from build123d import *

# Parameters (mm, degrees)
SKETCH1_R           = 20
BOSS_EXTRUDE1_DEPTH = 70
SKETCH2_R           = 15
CUT_EXTRUDE1_DEPTH  = 70
SKETCH3_R           = 2.5
CUT_EXTRUDE2_DEPTH  = 53


with BuildPart() as part:
    # Sketch1 → Boss-Extrude1 (new body)
    with BuildSketch(Plane.XY):
        Circle(SKETCH1_R)
    extrude(amount=BOSS_EXTRUDE1_DEPTH)

    # Sketch2 → Cut-Extrude1 (cut)
    with BuildSketch(Plane.XY.offset(70)):
        Circle(SKETCH2_R)
    extrude(amount=-CUT_EXTRUDE1_DEPTH, mode=Mode.SUBTRACT)

    # Sketch3 → Cut-Extrude2 (cut)
    with BuildSketch(Plane(origin=(20, 0, 0), x_dir=(0, 0, -1), z_dir=(1, 0, 0))):
        with Locations((-25, 0)):
            Circle(SKETCH3_R)
    extrude(amount=-CUT_EXTRUDE2_DEPTH, mode=Mode.SUBTRACT)


solid = part.part
The listing builds one solid part. Answer for the finished solid, in the listing's coordinates (mm). Coordinates: 2 decimals unless noted, no trailing zeros. Write each loop counter-clockwise with the first axis right and the second up, starting at its lowest first coordinate (ties: lowest second). Pieces come first, ordered by that corner, then holes. Notation, with made-up numbers: M 55,50.5 L 91,50.5 A15 cw 91,66.5 Z; hole C 52,18.25 d8. An arc over 180 degrees is marked long. Write each question's results on one line, items separated by ' | '.
Item 1: For a pull along Z with two mould halves and no side action, classify faces 1 (the face through (-17.4, 0.1, 27.5)), 2 (the face through (17.4, 0.1, 27.5)), 3 (the face through (3, 15, 70)), 4 (the face through (19.076, 6.007, 34.51)) as released by +Z, released by -Z, zero draft, split by the parting line, or undercut.
Answer below:
face 1: undercut | face 2: undercut | face 3: released by +Z | face 4: zero draft
Item 2: The part is cut by section B-B on y = 0. Determine the outline of the cut face in (x, z).
Answer below:
outline: M -20,0 L -15,0 L -15,22.5 L -20,22.5 Z; M -20,27.5 L -15,27.5 L -15,70 L -20,70 Z; M 15,0 L 20,0 L 20,22.5 L 15,22.5 Z; M 15,27.5 L 20,27.5 L 20,70 L 15,70 Z
Item 3: The part is cut by section C-C on x = 12. Determine the outline of the cut face in (y, z).
Answer below:
outline: M -16,0 L -9,0 L -9,70 L -16,70 Z; M 9,0 L 16,0 L 16,70 L 9,70 Z
Item 4: The part is cut by section A-A on x = 0. Determine the outline of the cut face in (y, z).
Answer below:
outline: M -20,0 L -15,0 L -15,70 L -20,70 Z; M 15,0 L 20,0 L 20,70 L 15,70 Z
Item 5: The part is cut by section D-D on y = -16. Determine the outline of the cut face in (x, z).
Answer below:
outline: M -12,0 L 12,0 L 12,70 L -12,70 Z
Item 6: Consider probe 1 along Z at (x, y) = (16, 0); probe 2 along Y at (x, z) = (-7, 51) (1 decimal); probe 3 along X at (y, z) = (10, 18.5). Determine where each line is inside the solid, lowest interval first. Write a range as [from, to].
Answer below:
probe 1: [0, 22.5], [27.5, 70] | probe 2: [-18.7, -13.3], [13.3, 18.7] | probe 3: [-17.32, -11.18], [11.18, 17.32]
Item 7: Given P1, Ø1.5, axis at x = 6, y = -15.5, coming from the -Z side; P2, Ø3, axis at y = 0, z = 25, coming from the -X side; P3, Ø3, axis at x = 3, z = 48, coming from the -Y side; P4, Ø6, axis at x = 0, z = 61.5, coming from the +Y side, each flat-ended and moving along its own axis, determine where each tip first touches the part or whether it passes through.
Answer below:
P1: z = 0 | P2: through | P3: y = -19.94 | P4: y = 20
